Work out the finished part from the listing and answer in its coordinate system (mm). Face numbers are marked on the shaded views. A direction names the side the tool comes from. Give positions to 0.01 mm unless a question says otherwise; leave off trailing zeros. Write each loop counter-clockwise with the first axis right and the second up, starting at its lowest first coordinate (ties: lowest second). Pieces come first, ordered by that corner, then holes. Notation, with made-up numbers: (-17, 63) -> (31, 63) arc R28 cw to (31, 91) -> close; hole circle Ø10 at (40, -20). An arc over 180 degrees is marked (long way). Use a Markdown table: item, result. Add a question column.
Q1. Section C-C, the plane x = 20.5 is taken. Give the vertices of the cut face in (y, z).
Q2. Section A-A, the plane x = 2 is taken. Give the vertices of the cut face in (y, z), plus the area to 3 significant figures.
Q3. Each of these flat-tipped pins is pushed along its axis until it touches: pin 1 Ø2 at (y, z) = (-3, 97) entering from -X; pin 2 Ø1 at (x, z) = (4, 103) entering from +Y; pin 3 Ø2 at (x, z) = (2, 34.5) entering from +Y; pin 4 Ø8.5 at (x, z) = (14, 87) entering from -Y. Where does it stop, or does it pass through?
Q4. Section B-B, the plane z = 34.5 is taken. Give the vertices of the cut face in (x, y).
Q5. For the marked faces 1 and 2, determine the directions among +Z, -Z, +X, -X, +Y, -Y from which every point of the face is accessible in a straight line to the end or side of a thin tool.
Q6. Consider line 1 (Y direction, x = 24, z = 93); line 2 (X direction, y = -0.8, z = 60); line 3 (X direction, y = -1, z = 26.5). Determine where each line is inside the solid, lowest interval first.
from build123d import *

# Parameters (mm, degrees)
BOSS_EXTRUDE1_DEPTH = 171
SKETCH2_R           = 1.25
CUT_EXTRUDE1_DEPTH  = 50
SKETCH3_R           = 1.25
CUT_EXTRUDE2_DEPTH  = 50
CUT_EXTRUDE3_DEPTH  = 2
LPATTERN1_COUNT     = 7
LPATTERN1_PITCH     = 25.5
SKETCH5_W           = 58.422821226
SKETCH5_H           = 32.27704233
CUT_EXTRUDE4_DEPTH  = 36


with BuildPart() as part:
    # Sketch1 → Boss-Extrude1 (new body)
    with BuildSketch(Plane.XY):
        Polygon((0, 0), (32.09, 0), (33.178500502, -6.66165645), (29.624787969, -6.61699683), (28.739662203, -1.2), (0, -1.2), align=None)
    extrude(amount=BOSS_EXTRUDE1_DEPTH)

    # Sketch2 → Cut-Extrude1 (cut)
    with BuildSketch(Plane(origin=(0, 0, 0), x_dir=(1, 0, 0), z_dir=(0, 1, 0))):
        with Locations(Location((2, -9, 0), (0, 0, 270))):
            Circle(SKETCH2_R)
    cut_extrude1 = extrude(amount=-CUT_EXTRUDE1_DEPTH, mode=Mode.SUBTRACT)

    # Sketch3 → Cut-Extrude2 (cut)
    with BuildSketch(Plane(origin=(31.255513263, 5.107084422, 0), x_dir=(0, 0, -1), z_dir=(0.9869120666582158, 0.16125933363501674, 0))):
        with Locations(Location((-9, -8.674812016, 0), (0, 0, 90))):
            Circle(SKETCH3_R)
    cut_extrude2 = extrude(amount=-CUT_EXTRUDE2_DEPTH, mode=Mode.SUBTRACT)

    # Sketch4 → Cut-Extrude3 (cut)
    with BuildSketch(Plane(origin=(27.801321029, 4.542676754, 0), x_dir=(0, 0, 1), z_dir=(-0.9869120666582157, -0.1612593336350174, 0))):
        Polygon((7.816431948, -6.624812016), (6.632863896, -8.674812016), (7.816431948, -10.724812016), (10.183568052, -10.724812016), (11.367136104, -8.674812016), (10.183568052, -6.624812016), align=None)
    cut_extrude3 = extrude(amount=-CUT_EXTRUDE3_DEPTH, mode=Mode.SUBTRACT)

    # LPattern1: Cut-Extrude1, Cut-Extrude2, Cut-Extrude3 ×7
    with Locations(*[(0, 0, i * LPATTERN1_PITCH) for i in range(1, LPATTERN1_COUNT)]):
        add(cut_extrude1, mode=Mode.SUBTRACT)
        add(cut_extrude2, mode=Mode.SUBTRACT)
        add(cut_extrude3, mode=Mode.SUBTRACT)

    # Sketch5 → Cut-Extrude4 (cut)
    with BuildSketch(Plane.XY.offset(171)):
        with Locations((17.719091417, -1.694811413)):
            Rectangle(SKETCH5_W, SKETCH5_H)
    extrude(amount=-CUT_EXTRUDE4_DEPTH, mode=Mode.SUBTRACT)


solid = part.part
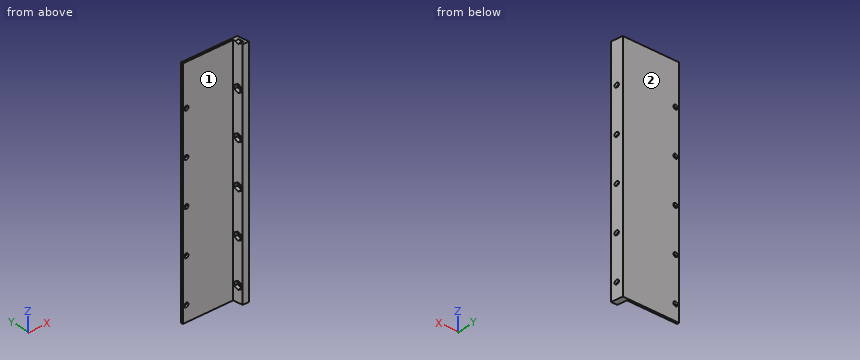
Result set:
| question | item | result |
|---|---|---|
| 1 | outline | (-1.2, 0) -> (0, 0) -> (0, 135) -> (-1.2, 135) -> close |
| 2 | outline | (-1.2, 0) -> (0, 0) -> (0, 7.75) -> (-1.2, 7.75) -> close; (-1.2, 10.25) -> (0, 10.25) -> (0, 33.25) -> (-1.2, 33.25) -> close; (-1.2, 35.75) -> (0, 35.75) -> (0, 58.75) -> (-1.2, 58.75) -> close; (-1.2, 61.25) -> (0, 61.25) -> (0, 84.25) -> (-1.2, 84.25) -> close; (-1.2, 86.75) -> (0, 86.75) -> (0, 109.75) -> (-1.2, 109.75) -> close; (-1.2, 112.25) -> (0, 112.25) -> (0, 135) -> (-1.2, 135) -> close |
| 2 | area | 147 mm2 |
| 3 | pin 1 | stops at x = 28.87 |
| 3 | pin 2 | stops at y = 0 |
| 3 | pin 3 | passes through |
| 3 | pin 4 | stops at y = -1.2 |
| 4 | outline | (0, -1.2) -> (0.75, -1.2) -> (0.75, 0) -> (0, 0) -> close; (3.25, -1.2) -> (28.74, -1.2) -> (28.87, -2) -> (30.84, -1.67) -> (30.97, -2.46) -> (32.45, -2.22) -> (32.09, 0) -> (3.25, 0) -> close; (29.53, -6.04) -> (29.62, -6.62) -> (33.18, -6.66) -> (32.86, -4.69) -> (31.38, -4.93) -> (31.5, -5.72) -> close |
| 5 | face 1 | +Z, -Z, -X, -Y |
| 5 | face 2 | +Z, -Z, +X, -X, +Y |
| 6 | line 1 | y = -1.2 to 0 |
| 6 | line 2 | x = 0 to 0.75, 3.25 to 32.22 |
| 6 | line 3 | x = 0 to 32.25 |
